from build123d import *

# Parameters (mm, degrees)
SKETCH1_W           = 21.5
SKETCH1_H           = 11.6
BOSS_EXTRUDE1_DEPTH = 13
SKETCH2_R           = 1
BOSS_EXTRUDE2_DEPTH = 1.2
SKETCH3_W           = 21.5
SKETCH3_H           = 11.6
BOSS_EXTRUDE3_DEPTH = 3.6
BOSS_EXTRUDE4_DEPTH = 2
SKETCH5_R           = 1.9
BOSS_EXTRUDE5_DEPTH = 2.8


with BuildPart() as part:
    # Sketch1 → Boss-Extrude1 (new body)
    with BuildSketch(Plane(origin=(0, 0, 0), x_dir=(1, 0, 0), z_dir=(0, 1, 0))):
        Rectangle(SKETCH1_W, SKETCH1_H)
    extrude(amount=BOSS_EXTRUDE1_DEPTH)

    # Sketch2 → Boss-Extrude2 (add)
    with BuildSketch(Plane(origin=(0, 13, 0), x_dir=(1, 0, 0), z_dir=(0, 1, 0))):
        Polygon((-10.75, 5.8), (-14.75, 3.75), (-14.75, -3.75), (-10.75, -5.8), (10.75, -5.8), (14.75, -3.75), (14.75, 3.75), (10.75, 5.8), align=None)
        with Locations(Location((-13, 0, 0), (0, 0, 270))):
            Circle(SKETCH2_R, mode=Mode.SUBTRACT)
        with Locations(Location((13, 0, 0), (0, 0, 90))):
            Circle(SKETCH2_R, mode=Mode.SUBTRACT)
    extrude(amount=BOSS_EXTRUDE2_DEPTH)

    # Sketch3 → Boss-Extrude3 (add)
    with BuildSketch(Plane(origin=(0, 14.2, 0), x_dir=(1, 0, 0), z_dir=(0, 1, 0))):
        Rectangle(SKETCH3_W, SKETCH3_H)
    extrude(amount=BOSS_EXTRUDE3_DEPTH)

    # Sketch4 → Boss-Extrude4 (add)
    with BuildSketch(Plane(origin=(0, 17.8, 0), x_dir=(1, 0, 0), z_dir=(0, 1, 0))):
        with BuildLine():
            ThreePointArc((0.103333333, 2.846721311), (-10.75, 0), (0.103333333, -2.846721311))
            ThreePointArc((0.103333333, -2.846721311), (4.05, 0), (0.103333333, 2.846721311))
        make_face()
    extrude(amount=BOSS_EXTRUDE4_DEPTH)

    # Sketch5 → Boss-Extrude5 (add)
    with BuildSketch(Plane(origin=(0, 19.8, 0), x_dir=(1, 0, 0), z_dir=(0, 1, 0))):
        with Locations(Location((-4.95, 0, 0), (0, 0, 270))):
            Circle(SKETCH5_R)
    extrude(amount=BOSS_EXTRUDE5_DEPTH)


solid = part.part
For this review, take the finished solid that the model builds, in its own axes (mm). A direction names the side the tool comes from. Give positions to 0.01 mm unless a question says otherwise; leave off trailing zeros. Loops run counter-clockwise (first coordinate to the right, second up) from the corner with the lowest first, then second, coordinate; pieces in that order, holes last. Notation, with made-up numbers: M -9,32 L 32,32 A26 ccw 32,70 Z; hole C -9,-6.75 d10. An arc over 180 degrees is marked long. Answer as a JSON object with one key per item and string values. Group by question number.
Q1. Add section A-A on x = 1.05. Give the boundary of the cut face in (y, z).
Q2. Mouldability with a two-part tool opening along X and no side actions: class faces 1 (the flat face through (12.7, 13.6, 4.8)), 2 (the flat face through (-10, 17.8, 4)), 3 (the cylindrical face through (14, 14, 0)) as +X half, -X half, draft (parallel to the pull), parting line (faces both ways), or undercut.
Q3. Add section C-C on z = 0.5. Give the number of separate pieces and of enclosed holes in the cut face, and give its area (3 significant figures).
Q4. Add section B-B on x = 13. Give the boundary of the cut face in (y, z), and give its area (3 significant figures).
Q5. Add section D-D on y = 9.5. Give the boundary of the cut face in (x, z), and give its area (3 significant figures).
Q6. Insertion check: P1, Ø4.5, axis at x = -13.5, z = -2, coming from the +Y side; P2, Ø1.1, axis at y = 17, z = 2, coming from the +X side; P3, Ø3.5, axis at x = 5, z = 2, coming from the +Y side; P4, Ø1.6, axis at x = 13, z = 0, coming from the -Y side. Each pin has a flat end and moves straight along its axis. Give the tip position at first contact, or say it passes through.
Q7. Tool access review of faces 4 (the flat face through (-10, 17.8, -4)), 5 (the flat face through (10.75, 6, 0)), 6 (the flat face through (-10.75, 6, 0)), 7 (the flat face through (-3, 19.8, -1)), 8 (the flat face through (-12.8, 14.2, 1.2)): name each direction out of +Z, -Z, +X, -X, +Y, -Y from which nothing blocks a thin tool from reaching the whole face with its end or side.
Q8. For probe 1 along X at (y, z) = (13.95, 0); probe 2 along Y at (x, z) = (-8.25, -1.75); probe 3 along X at (y, z) = (15.5, 0.25), list the stretches that pass through material, from the lowest coordinate up. Write a range as [from, to].
Checked values:
{
 "1": {"outline": "M 0,-5.8 L 17.8,-5.8 L 17.8,-3 L 19.8,-3 L 19.8,3 L 17.8,3 L 17.8,5.8 L 0,5.8 Z"},
 "2": {"face 1": "+X half", "face 2": "draft", "face 3": "undercut"},
 "3": {"separate pieces": "3", "enclosed holes": "0", "area": "428 mm²"},
 "4": {"outline": "M 13,-4.65 L 14.2,-4.65 L 14.2,-1 L 13,-1 Z; M 13,1 L 14.2,1 L 14.2,4.65 L 13,4.65 Z", "area": "8.75 mm²"},
 "5": {"outline": "M -10.75,-5.8 L 10.75,-5.8 L 10.75,5.8 L -10.75,5.8 Z", "area": "249 mm²"},
 "6": {"P1": "y = 14.2", "P2": "x = 10.75", "P3": "y = 19.8", "P4": "through"},
 "7": {"face 4": "-Z, -X, +Y", "face 5": "+Z, -Z, +X, -Y", "face 6": "+Z, -Z, -X, -Y", "face 7": "+Y", "face 8": "+Z, -Z, -X, +Y"},
 "8": {"probe 1": "[-14.75, -14], [-12, 12], [14, 14.75]", "probe 2": "[0, 19.8]", "probe 3": "[-10.75, 10.75]"}
}
